Geometry check sheet. Reference: the model listing, model coordinates, mm. Face numbers are marked on the shaded views. Coordinates: 2 decimals unless noted, no trailing zeros. Loops run counter-clockwise (first coordinate to the right, second up) from the corner with the lowest first, then second, coordinate; pieces in that order, holes last.
from build123d import *

# Parameters (mm, degrees)
F1_DEPTH = 40
F2_D     = 28
F4_D     = 5.5
F4_DEPTH = 20
F4_TIP   = 1.6523667023


with BuildPart() as f1:
    # F0 (on Front) → F1 (new body)
    with BuildSketch(Plane.XZ):
        Polygon((26, 22.7809774678), (-26, 22.7809774678), (-26, -7.2190225322), (-14, -17.2190225322), (14, -17.2190225322), (26, -7.2190225322), align=None)
    extrude(amount=F1_DEPTH)

    # F2 (through all)
    with Locations(Plane(origin=(0, 0, 0), x_dir=(1, 0, 0), z_dir=(0, 1, 0))):
        with Locations((0, -2.7809774678)):
            Hole(F2_D / 2)

    # F4
    with Locations(Plane.XY.offset(22.7809774678)):
        with Locations((-20, -8), (-20, -32), (20, -32), (20, -8)):
            Hole(F4_D / 2, depth=F4_DEPTH)
            with Locations((0, 0, -(F4_DEPTH + F4_TIP / 2))):  # 118° drill point
                Cone(0, F4_D / 2, F4_TIP, mode=Mode.SUBTRACT)


solid = f1.part
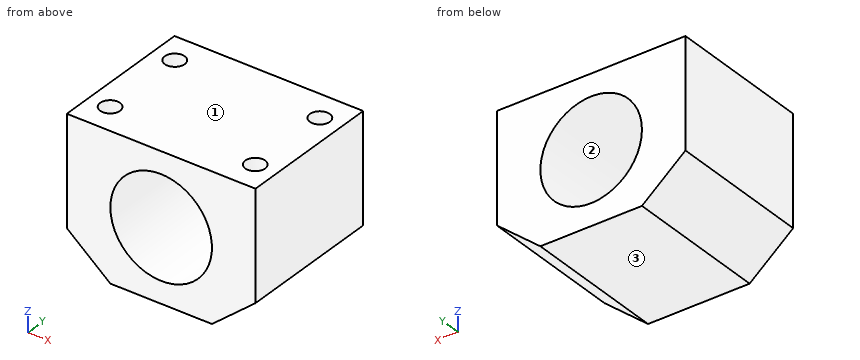
1) Mould release check, pull along Z, two halves, no side actions. Record for the marked faces 1, 2 and 3: +Z half, -Z half, draft (parallel to the pull), parting line (faces both ways), or undercut.
Data:
face 1: +Z half
face 2: undercut
face 3: -Z half
2) Section check B-B on y = -22. Record the cut outline in (x, z), and give its area (3 significant figures).
Data:
outline: (-26, -7.22) - (-14, -17.22) - (14, -17.22) - (26, -7.22) - (26, 22.78) - (-26, 22.78) - close; hole circle Ø28 at (0, 2.78)
area: 1,340 mm2
3) Material ranges on probe 1 along Y at (x, z) = (-20, 14); probe 2 along X at (y, z) = (-32, 15); probe 3 along X at (y, z) = (-8, 17.5), recorded low to high.
Data:
probe 1: y = -40 to -34.75, -29.25 to -10.75, -5.25 to 0
probe 2: x = -26 to -22.75, -17.25 to -6.83, 6.83 to 17.25, 22.75 to 26
probe 3: x = -26 to -22.75, -17.25 to 17.25, 22.75 to 26
4) Depth check by flat-ended pin: pin 1 (6.5 mm diameter, centred on x = -20, y = -32, fed in from -Z); pin 2 (4.5 mm diameter, centred on x = -20, y = -8, fed in from -Z); pin 3 (12 mm diameter, centred on x = -15, y = -11, fed in from -Z); pin 4 (9 mm diameter, centred on x = 20, y = -32, fed in from -Z). Enter the tip coordinate at first touch or a pass-through.
Data:
pin 1: stops at z = -14.93
pin 2: stops at z = -14.09
pin 3: stops at z = -17.22
pin 4: stops at z = -15.97
5) Section check C-C on x = -7. Record the cut outline in (y, z), and give its area (3 significant figures).
Data:
outline: (-40, -17.22) - (0, -17.22) - (0, -9.34) - (-40, -9.34) - close; (-40, 14.91) - (0, 14.91) - (0, 22.78) - (-40, 22.78) - close
area: 630 mm2
6) Section check A-A on x = 0. Record the cut outline in (y, z).
Data:
outline: (-40, -17.22) - (0, -17.22) - (0, -11.22) - (-40, -11.22) - close; (-40, 16.78) - (0, 16.78) - (0, 22.78) - (-40, 22.78) - close
